Autodesk Inventor part; units mm, degrees
ref_plane "YZ Plane" through (0, 0, 0) normal (1, 0, 0) x (0, 1, 0)
ref_plane "XZ Plane" through (0, 0, 0) normal (0, 1, 0) x (-1, 0, 0)
ref_plane "XY Plane" through (0, 0, 0) normal (0, 0, 1) x (1, 0, 0)
sketch "Sketch1" plane through (0, 0, 0) normal (0, 1, 0) x (-1, 0, 0)
  arc A0 (8.5, 13.7081) -> (11.5, 13.7081) centre (10, 10) ccw
  line L0 (8.5, 20) -> (8.5, 13.7081)
  line L1 (11.5, 20) -> (11.5, 13.7081)
  line L2 (10, 20) -> (10, 18.7339)
  line L3 (20, 20) -> (10, 20)
  line L4 (8.5, 20) -> (0, 20)
  line L5 (0, 20) -> (0, 0)
  line L6 (0, 0) -> (20, 0)
  line L7 (20, 0) -> (20, 20)
  arc A1 (68.5, 13.7081) -> (71.5, 13.7081) centre (70, 10) ccw
  line L8 (68.5, 20) -> (68.5, 13.7081)
  line L9 (71.5, 20) -> (71.5, 13.7081)
  line L10 (70, 20) -> (70, 18.3732)
  line L11 (80, 20) -> (70, 20)
  line L12 (68.5, 20) -> (60.9559, 20)
  line L13 (60.9559, 20) -> (60.9559, 0)
  line L14 (60.9559, 0) -> (80, 0)
  line L15 (80, 0) -> (80, 20)
  line L16 (60.9559, 0) -> (20, 0)
  line L17 (20, 0) -> (20, 20)
  line L18 (20, 20) -> (60.9559, 20)
  line L19 (60.9559, 20) -> (60.9559, 0)
  dimension "d2" = 8
  dimension "d7" = 1.5
  dimension "d8" = 1.5
  dimension "d16" = 10
  dimension "d17" = 8
  dimension "d18" = 1.5
  dimension "d19" = 1.5
  dimension "d20" = 10
  dimension "d22" = 80
  dimension "d23" = 10
  dimension "d24" = 0
  dimension "d25" = 60
  dimension "d26" = 20
  dimension "d27" = 20
  dimension "d28" = 20
  dimension "d29" = 20
  dimension "d30" = 10
  dimension "d31" = 10
  dimension "d32" = 20
extrude "Extrusion1" add sketch "Sketch1" along normal blind 36
sketch "Sketch5" plane through (-80, 0, 0) normal (-1, 0, 0) x (0, 0, 1)
  line L0 (20, 0) -> (20, 36)
  line L1 (20, 36) -> (-15, 36)
  line L2 (-15, 6) -> (20, 6)
  line L3 (20, 6) -> (20, 36)
  line L4 (-15, 36) -> (-15, 26.6522)
  line L5 (-15, 15.4718) -> (-15, 6)
  line L6 (0, 0) -> (0, 36)
  line L7 (0, 0) -> (0, 36)
  line L8 (0, 6) -> (0, 36)
  arc A0 (-15, 15.4718) -> (-15, 26.6522) centre (-10, 21.062) ccw
  dimension "d40" = 30
  dimension "d41" = 35
  dimension "d45" = 20
  dimension "d85" = 15
  dimension "d86" = 5
  dimension "d87" = 15
extrude "Extrusion5" add sketch "Sketch5" against normal blind 80 contours L2 L5 A0 L4 L1 L6
sketch "Sketch13" plane through (0, 36, 0) normal (0, 1, 0) x (1, 0, 0)
  line L0 (-80, -20) -> (-80, 15)
  line L1 (-80, -20) -> (-71.5, -20)
  line L2 (-71.5, -20) -> (-71.5, -13.7081)
  arc A0 (-68.5, -13.7081) -> (-71.5, -13.7081) centre (-70, -10) ccw
  line L3 (-68.5, -13.7081) -> (-68.5, -20)
  line L4 (-68.5, -20) -> (-11.5, -20)
  line L5 (-11.5, -20) -> (-11.5, -13.7081)
  arc A1 (-8.5, -13.7081) -> (-11.5, -13.7081) centre (-10, -10) ccw
  line L6 (-8.5, -13.7081) -> (-8.5, -20)
  line L7 (-8.5, -20) -> (0, -20)
  line L8 (0, -20) -> (0, 15)
  line L9 (-80, 15) -> (0, 15)
  point P0 (0, 0)
extrude "Extrusion11" cut sketch "Sketch13" against normal blind 1
equation "\"d2\" = RodDiameter"
equation "\"d17\" = d2"
equation "\"RodDiameter\" = 8"
equation "\"VerticalBearingOD\" = 16"
equation "\"PrintingClearance\" = 0.2"
equation "\"d21\" = 8"
properties part number "GantryHolder"
Input: part model. Units: mm. Frame: model coordinates. A direction names the side the tool comes from. Coordinates: 2 decimals unless noted, no trailing zeros. Write each loop counter-clockwise with the first axis right and the second up, starting at its lowest first coordinate (ties: lowest second). Pieces come first, ordered by that corner, then holes.
1) Section B-B on z = -10. Output: boundary loops of the cut face in (x, y), and give its area (3 significant figures).
2) Mould query, pull axis Z, two halves, no side actions, for faces 1 (the flat face through (-68.5, 17, 17)), 2 (the cylindrical face through (-10, 17, 6)), 3 (the flat face through (-41, 31, -15)). Classes: pulls with the +Z half, pulls with the -Z half, needs draft (parallel to the pull), parting line crosses it, or undercut.
3) Section A-A on z = 17. Output: boundary loops of the cut face in (x, y).
4) Pin query (flat end, axial travel): pin 1 Ø6 at (x, y) = (-25, 20.5) entering from -Z; pin 2 Ø6.5 at (x, y) = (-41, 2) entering from -Z; pin 3 Ø16.5 at (x, z) = (-57, -9) entering from -Y. Return the tip coordinate at first contact, or that it passes through.
5) Section D-D on x = -65. Output: boundary loops of the cut face in (y, z).
6) Material intervals for line 1 along X through (y, z) = (22, 16); line 2 along X through (y, z) = (14.5, 10); line 3 along Y through (x, z) = (-34, -10), sorted ascending.
7) Section C-C on y = 4. Output: boundary loops of the cut face in (x, z).
8) Set-up query: faces 4 (the cylindrical face through (-70, 17, 6)), 5 (the flat face through (-41, 6, -8)), 6 (the flat face through (-8.5, 17, 17)). Return all of +Z, -Z, +X, -X, +Y, -Y with unobstructed straight access to the full face (end or side cutting, diameter ignored); none if empty.
Check result:
1. outline: (-80, 6) - (0, 6) - (0, 13.56) - (-80, 13.56) - close; (-80, 28.56) - (0, 28.56) - (0, 35) - (-80, 35) - close
1. area: 1,120 mm2
2. face 1: needs draft
2. face 2: undercut
2. face 3: pulls with the -Z half
3. outline: (-80, 0) - (-71.5, 0) - (-71.5, 35) - (-80, 35) - close; (-68.5, 0) - (-11.5, 0) - (-11.5, 35) - (-68.5, 35) - close; (-8.5, 0) - (0, 0) - (0, 35) - (-8.5, 35) - close
4. pin 1: stops at z = -3.4
4. pin 2: stops at z = 0
4. pin 3: stops at y = 6
5. outline: (0, 0) - (6, 0) - (6, -15) - (15.47, -15) arc R7.5 cw (long way) to (26.65, -15) - (35, -15) - (35, 20) - (0, 20) - close
6. line 1: x = -80 to -71.5, -68.5 to -11.5, -8.5 to 0
6. line 2: x = -80 to -74, -66 to -14, -6 to 0
6. line 3: y = 6 to 13.56, 28.56 to 35
7. outline: (-80, 0) - (0, 0) - (0, 20) - (-8.5, 20) - (-8.5, 13.71) arc R4 cw (long way) to (-11.5, 13.71) - (-11.5, 20) - (-68.5, 20) - (-68.5, 13.71) arc R4 cw (long way) to (-71.5, 13.71) - (-71.5, 20) - (-80, 20) - close
8. face 4: +Y, -Y
8. face 5: -Z, +X, -X, -Y
8. face 6: +Z, +Y, -Y
